The listing builds one solid part. Answer for the finished solid, in the listing's coordinates (mm). Round coordinates to 2 decimals unless told otherwise and drop trailing zeros. Loops run counter-clockwise (first coordinate to the right, second up) from the corner with the lowest first, then second, coordinate; pieces in that order, holes last. Notation, with made-up numbers: (-27, 5.25) -> (-17, 5.25) arc R29 cw to (-17, 37.25) -> close; hole circle Ø11 at (87.5, -27.75). An arc over 180 degrees is marked (long way). Use a Markdown table: item, result. Add a question column.
Q1. Consider line 1 (X direction, y = 4, z = 380); line 2 (Y direction, x = -2.5, z = 378); line 3 (Y direction, x = -6.25, z = 199.5). Determine where each line is inside the solid, lowest interval first.
Q2. Given pin 1 Ø5.5 at (x, z) = (0, 80) entering from +Y, flat-ended and moving along its own axis, determine where the tip first touches the part or whether it passes through.
Q3. Section A-A on z = 409.5 is taken. Give the vertices of the cut face in (x, y).
Autodesk Inventor part; units mm, degrees
ref_plane "YZ Plane" through (0, 0, 0) normal (1, 0, 0) x (0, 1, 0)
ref_plane "XZ Plane" through (0, 0, 0) normal (0, 1, 0) x (-1, 0, 0)
ref_plane "XY Plane" through (0, 0, 0) normal (0, 0, 1) x (1, 0, 0)
sketch "Sketch1" plane through (0, 0, 0) normal (0, 0, 1) x (1, 0, 0)
  line L0 (0, 0) -> (0, 17.5) construction
  line L1 (0, 0) -> (-10, 0)
  line L2 (0, 0) -> (10, 0)
  line L3 (-10, 0) -> (-10, 4.6)
  line L4 (-10, 4.6) -> (-6.1, 8.5)
  line L5 (-6.1, 8.5) -> (-6.1, 9)
  line L6 (-6.1, 9) -> (-10, 12.9)
  line L7 (-10, 12.9) -> (-10, 15.4)
  line L8 (-10, 15.4) -> (-7.9, 17.5)
  line L9 (-7.9, 17.5) -> (0, 17.5)
  line L10 (10, 0) -> (10, 4.6)
  line L11 (10, 4.6) -> (6.1, 8.5)
  line L12 (6.1, 8.5) -> (6.1, 9)
  line L13 (6.1, 9) -> (10, 12.9)
  line L14 (10, 12.9) -> (10, 15.4)
  line L15 (10, 15.4) -> (7.9, 17.5)
  line L16 (7.9, 17.5) -> (0, 17.5)
  dimension "d0" = 17.5
  dimension "d1" = 20
  dimension "d2" = 4.6
  dimension "d3" = 8.5
  dimension "d8" = 135
  dimension "d9" = 0.5
  dimension "d10" = 135
  dimension "d11" = 2.5
extrude "Extrusion1" add sketch "Sketch1" along normal blind 800
sketch "Sketch2" plane through (0, 0, 0) normal (0, 1, 0) x (-1, 0, 0)
  line L0 (0, 0) -> (0, 20) construction
  line L1 (0, 20) -> (0, 80) construction
  circle A0 centre (0, 20) radius 4.75
  circle A1 centre (0, 20) radius 3
  dimension "d14" = 20
  dimension "d15" = 60
  dimension "d16" = 9.5
  dimension "d17" = 6
extrude "Extrusion2" cut sketch "Sketch2" along normal through all contours A1
extrude "Extrusion3" cut sketch "Sketch2" against normal blind 8.5 from surface at 17.5
pattern_linear "Rectangular Pattern1" count 14 spacing 60 along (0, 0, 1) of "Extrusion2", "Extrusion3"
properties part number "HGR20 500mm"
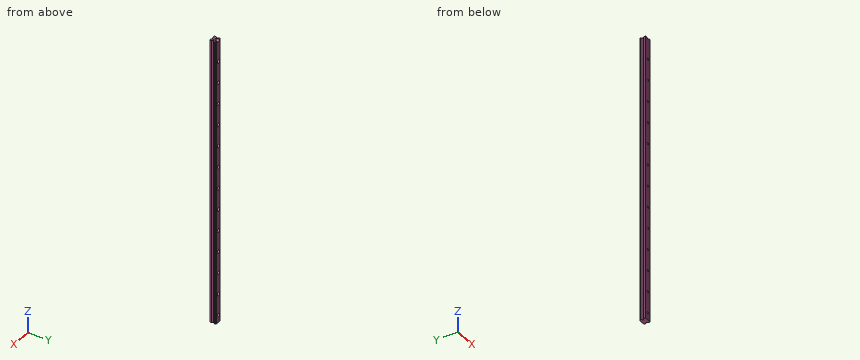
Checked values:
| question | item | result |
|---|---|---|
| 1 | line 1 | x = -10 to -3, 3 to 10 |
| 1 | line 2 | y = 0 to 9 |
| 1 | line 3 | y = 0 to 8.35, 9.15 to 17.5 |
| 2 | pin 1 | passes through |
| 3 | outline | (-10, 0) -> (10, 0) -> (10, 4.6) -> (6.1, 8.5) -> (6.1, 9) -> (10, 12.9) -> (10, 15.4) -> (7.9, 17.5) -> (-7.9, 17.5) -> (-10, 15.4) -> (-10, 12.9) -> (-6.1, 9) -> (-6.1, 8.5) -> (-10, 4.6) -> close |
